from build123d import *

# Parameters (mm, degrees)
BOSS_EXTRUDE1_DEPTH = 5
SKETCH2_R           = 1.7
CUT_EXTRUDE1_DEPTH  = 10


with BuildPart() as part:
    # Sketch1 → Boss-Extrude1 (new body)
    with BuildSketch(Plane(origin=(0, 0, 0), x_dir=(1, 0, 0), z_dir=(0, 1, 0))):
        Polygon((-82.5, 60), (-82.5, 65), (-77.5, 65), (-62.5, 65), (-62.5, 60), (-42.5, 60), (-42.5, 65), (-27.5, 65), (-27.5, 60), (-7.5, 60), (-7.5, 65), (7.5, 65), (7.5, 60), (27.5, 60), (27.5, 65), (42.5, 65), (42.5, 60), (62.5, 60), (62.5, 65), (77.5, 65), (82.5, 65), (82.5, 60), (82.5, 45), (77.5, 45), (77.5, 25), (82.5, 25), (82.5, 10), (77.5, 10), (77.5, -10), (82.5, -10), (82.5, -25), (77.5, -25), (77.5, -45), (82.5, -45), (82.5, -60), (82.5, -65), (77.5, -65), (62.5, -65), (62.5, -60), (42.5, -60), (42.5, -65), (27.5, -65), (27.5, -60), (7.5, -60), (7.5, -65), (-7.5, -65), (-7.5, -60), (-27.5, -60), (-27.5, -65), (-42.5, -65), (-42.5, -60), (-62.5, -60), (-62.5, -65), (-77.5, -65), (-82.5, -65), (-82.5, -60), (-82.5, -45), (-77.5, -45), (-77.5, -25), (-82.5, -25), (-82.5, -10), (-77.5, -10), (-77.5, 10), (-82.5, 10), (-82.5, 25), (-77.5, 25), (-77.5, 45), (-82.5, 45), align=None)
    extrude(amount=BOSS_EXTRUDE1_DEPTH)

    # Sketch2 → Cut-Extrude1 (cut)
    with BuildSketch(Plane(origin=(0, 5, 0), x_dir=(1, 0, 0), z_dir=(0, 1, 0))):
        with Locations(Location((-11.999998057, -11.999998057, 0), (0, 0, 270))):
            Circle(SKETCH2_R)
        with Locations(Location((-11.999998057, 11.999998057, 0), (0, 0, 270))):
            Circle(SKETCH2_R)
        with Locations(Location((11.999998057, 11.999998057, 0), (0, 0, 270))):
            Circle(SKETCH2_R)
        with Locations(Location((11.999998057, -11.999998057, 0), (0, 0, 270))):
            Circle(SKETCH2_R)
    extrude(amount=-CUT_EXTRUDE1_DEPTH, mode=Mode.SUBTRACT)


solid = part.part
Work out the finished part from the listing and answer in its coordinate system (mm). A direction names the side the tool comes from. Round coordinates to 2 decimals unless told otherwise and drop trailing zeros. Order: outer loops, then holes, each group sorted by start corner. A loop starts at its lowest first (then second) coordinate and runs counter-clockwise, first axis right, second up. Notation, with made-up numbers: M 13,-27.5 L 54,-27.5 A7 cw 54,-16.5 Z; hole C -18,53.25 d4. An arc over 180 degrees is marked long. Put each result on its own line as item: value. Start each with the question number.
Q1. For a pull along X with two mould halves and no side action, classify faces 6 (the flat face through (27.5, 2, 63)), 7 (the flat face through (82.5, 2, 17)), 8 (the flat face through (7.5, 2, -63)), 9 (the flat face through (-80, 2, -10)) as pulls with the +X half, pulls with the -X half, needs draft (parallel to the pull), parting line crosses it, or undercut.
Q2. Section B-B, the plane z = -4 is taken. Write down the section's boundary in (x, y), and give its area (3 significant figures).
Q3. Straight lines are drawn through the part: L1, parallel to X at y = 2.25, z = -1.5; L2, parallel to Z at x = -13, y = 1.15; L3, parallel to Z at x = -20, y = 1.85. For each, find the intervals that lie inside material, in ascending order. Write a range as [from, to].
Q4. A tool of negligible diameter and unlimited length cuts with its end or side. For faces 1 (the flat face through (-73, 2, 65)), 2 (the flat face through (52, 2, -60)), 3 (the flat face through (53, 2, 60)), 4 (the flat face through (80, 2, -10)), 5 (the flat face through (-80, 2, 25)), from which of +Z, -Z, +X, -X, +Y, -Y can it reach the whole face along a straight path? Write none if from no direction.
Q5. Flat-ended cylindrical pins translate along their axes: pin 1 (5 mm diameter, centred on x = 27.5, z = 47.5, fed in from -Y); pin 2 (1.5 mm diameter, centred on y = 2.5, z = 0, fed in from -X); pin 3 (1.5 mm diameter, centred on x = 18.5, y = 3.5, fed in from -Z). Find the tip coordinate at first contact, or state that the pin passes through.
Q6. Section C-C, the plane x = 24.5 is taken. Write down the section's boundary in (y, z).
Q7. Section A-A, the plane y = 1.15 is taken. Give the number of separate pieces and of enclosed holes in the cut face, and give its area (3 significant figures).
Findings below:
1. face 6: undercut
1. face 7: pulls with the +X half
1. face 8: undercut
1. face 9: needs draft
2. outline: M -77.5,0 L 77.5,0 L 77.5,5 L -77.5,5 Z
2. area: 775 mm^2
3. L1: x = [-77.5, 77.5]
3. L2: z = [-60, -13.37], [-10.63, 10.63], [13.37, 60]
3. L3: z = [-60, 60]
4. face 1: +Z, +X, -X, +Y, -Y
4. face 2: -Z, +Y, -Y
4. face 3: +Z, +Y, -Y
4. face 4: +X, +Y, -Y
4. face 5: -X, +Y, -Y
5. pin 1: stops at y = 0
5. pin 2: stops at x = -77.5
5. pin 3: stops at z = -60
6. outline: M 0,-60 L 5,-60 L 5,60 L 0,60 Z
7. separate pieces: 1
7. enclosed holes: 4
7. area: 20,000 mm^2
